Can you work these out from the model? Positions are in its coordinate system, mm. Coordinates: 2 decimals unless noted, no trailing zeros. Loops run counter-clockwise (first coordinate to the right, second up) from the corner with the lowest first, then second, coordinate; pieces in that order, holes last.
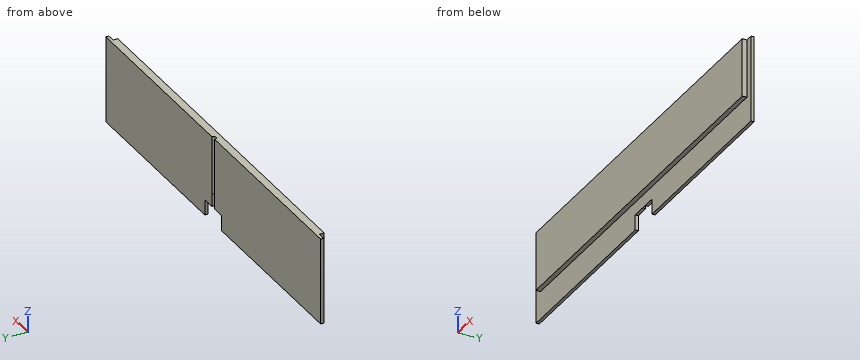
```python
from build123d import *

# Parameters (mm, degrees)
SKETCH074_W          = 245
SKETCH074_H          = 38
PAD035_DEPTH         = 3
PAD036_DEPTH         = 2
SKETCH087_R          = 1.75
POCKET037_DEPTH      = 18.251
POCKET037_DEPTH_BACK = 38.001


with BuildPart() as part:
    # Sketch074 → Pad035 (new body)
    with BuildSketch(Plane.XZ):
        with Locations((122.5, 19)):
            Rectangle(SKETCH074_W, SKETCH074_H)
    extrude(amount=PAD035_DEPTH)

    # Sketch075 → Pad036 (join)
    with BuildSketch(Plane.XZ):
        Polygon((-5, 38), (-5, -18.25), (112.5, -18.25), (112.5, -8.25), (132.5, -8.25), (132.5, -18.25), (250, -18.25), (250, 38), align=None)
    extrude(amount=-PAD036_DEPTH)

    # Sketch087 → Pocket037 (cut, two sides)
    with BuildSketch(Plane.XY) as pocket037_sk:
        with Locations((122.5, 2)):
            Circle(SKETCH087_R)
    extrude(amount=-POCKET037_DEPTH, mode=Mode.SUBTRACT)
    extrude(pocket037_sk.sketch, amount=POCKET037_DEPTH_BACK, mode=Mode.SUBTRACT)


solid = part.part
```
(1) I want a section at B-B on x = 19. Write out the boundary of the cut face in (y, z), then the cut area to 4 significant figures.
Check values:
outline: (-3, 0) - (0, 0) - (0, -18.25) - (2, -18.25) - (2, 38) - (-3, 38) - close
area: 226.5 mm2
(2) I'm going to push flat-ended pins straight in: pin 1 (0.9 mm diameter, centred on y = -2, z = 16, fed in from -X); pin 2 (1.6 mm diameter, centred on x = 127.5, y = 1, fed in from -Z); pin 3 (1.5 mm diameter, centred on x = 129, y = -1.5, fed in from -Z). Where does each tip first touch, or does it pass through?
Check values:
pin 1: stops at x = 0
pin 2: stops at z = -8.25
pin 3: stops at z = 0
(3) If I drill on probe 1 along X at (y, z) = (1.6, 25.5); probe 2 along X at (y, z) = (1.25, -12.5); probe 3 along X at (y, z) = (-1, 33), over which ranges is the centre line in solid material (lowest first)?
Check values:
probe 1: x = -5 to 120.8, 124.2 to 250
probe 2: x = -5 to 112.5, 132.5 to 250
probe 3: x = 0 to 245
(4) I want a section at A-A on z = 19. Write out the boundary of the cut face in (x, y), then the cut area to 3 significant figures.
Check values:
outline: (-5, 0) - (0, 0) - (0, -3) - (245, -3) - (245, 0) - (250, 0) - (250, 2) - (124.25, 2) arc R1.75 cw to (120.75, 2) - (-5, 2) - close
area: 1,240 mm2
(5) I want a section at C-C on y = -2.15. Write out the boundary of the cut face in (x, z), then the cut area to 3 significant figures.
Check values:
outline: (0, 0) - (245, 0) - (245, 38) - (0, 38) - close
area: 9,310 mm2
